```python
from build123d import *

# Parameters (mm, degrees)
F0_R     = 14.75
F1_DEPTH = 10
F3_DEPTH = 10


# Not quite as in the source:
# - a feature names something its author has since deleted; it is built from what else it names


with BuildPart() as f1:
    # F0 (on Top) → F1 (new body)
    with BuildSketch(Plane.XY):
        with BuildLine():
            ThreePointArc((0, 20), (5.8578643763, 5.8578643763), (20, 0))
            Line((20, 0), (97.5, 0))
            ThreePointArc((97.5, 0), (99.267766953, 0.732233047), (100, 2.5))
            Line((100, 2.5), (100, 37.5))
            ThreePointArc((100, 37.5), (99.267766953, 39.267766953), (97.5, 40))
            Line((97.5, 40), (20, 40))
            ThreePointArc((20, 40), (5.8578643763, 34.1421356237), (0, 20))
        make_face()
        with Locations((20, 20)):
            Circle(F0_R, mode=Mode.SUBTRACT)
    extrude(amount=F1_DEPTH)

    # F2 (on face) → F3 (join)
    with BuildSketch(Plane.XY.offset(10)):
        with BuildLine():
            ThreePointArc((22.5, 37.5), (21.767766953, 39.267766953), (20, 40))
            ThreePointArc((20, 40), (0, 20), (20, 0))
            ThreePointArc((20, 0), (21.767766953, 0.732233047), (22.5, 2.5))
            Line((22.5, 2.5), (22.5, 2.75))
            ThreePointArc((22.5, 2.75), (21.767766953, 4.517766953), (20, 5.25))
            ThreePointArc((20, 5.25), (5.25, 20), (20, 34.75))
            ThreePointArc((20, 34.75), (21.767766953, 35.482233047), (22.5, 37.25))
            Line((22.5, 37.25), (22.5, 37.5))
        make_face()
        with BuildLine():
            ThreePointArc((100, 37.5), (99.267766953, 39.267766953), (97.5, 40))
            ThreePointArc((97.5, 40), (95.732233047, 39.267766953), (95, 37.5))
            Line((95, 37.5), (95, 2.5))
            ThreePointArc((95, 2.5), (95.732233047, 0.732233047), (97.5, 0))
            ThreePointArc((97.5, 0), (99.267766953, 0.732233047), (100, 2.5))
            Line((100, 2.5), (100, 37.5))
        make_face()
    extrude(amount=F3_DEPTH)


solid = f1.part
```
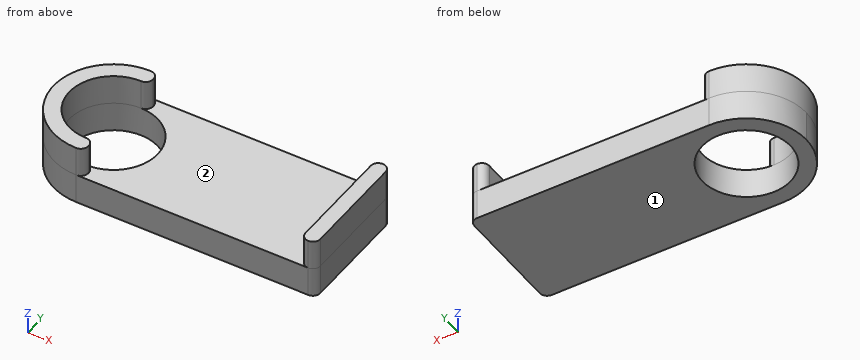
Design review of the part built by this model. Coordinates are the model's own, in mm. Face numbers are marked on the shaded views. Give positions to 0.01 mm unless a question says otherwise; leave off trailing zeros. Order: outer loops, then holes, each group sorted by start corner. A loop starts at its lowest first (then second) coordinate and runs counter-clockwise, first axis right, second up. Notation, with made-up numbers: (35, 18.25) - (79, 18.25) arc R16 cw to (79, 45.25) - close; hole circle Ø9 at (41.25, 71). An arc over 180 degrees is marked (long way). Use a Markdown table: item, result. Add a question column.
(1) Add section B-B on y = 27. Give the boundary of the cut face in (x, z) (3 decimals).
(2) Add section D-D on y = 15. Give the boundary of the cut face in (x, z), then the cut area to 3 significant figures.
(3) Add section A-A on z = 13. Give the boundary of the cut face in (x, y), then the cut area to 3 significant figures.
(4) Wall thickness on probe 1 along Y at (x, z) = (20, 4.5); probe 2 along X at (y, z) = (20, 4.25); probe 3 along Z at (x, y) = (82, 21): over which ranges is each line inside the solid? List them lowest first. Write a range as [from, to].
(5) Add section C-C on x = 37.5. Give the boundary of the cut face in (y, z).
(6) Clearance check with flat-ended pins moving along their axes: P1, Ø5, axis at y = 17, z = 15, coming from the -X side; P2, Ø8, axis at x = 52, z = 16, coming from the +Y side; P3, Ø12, axis at y = 29.5, z = 15.5, coming from the -X side; P4, Ø12, axis at x = 71.5, y = 21.5, coming from the +Z side. State where each tip first meets the part, or that it passes through.
(7) Mouldability with a two-part tool opening along X and no side actions: class the marked faces 1 and 2 as +X half, -X half, draft (parallel to the pull), parting line (faces both ways), or undercut.
Report:
| question | item | result |
|---|---|---|
| 1 | outline | (1.265, 0) - (7.017, 0) - (7.017, 20) - (1.265, 20) - close; (32.983, 0) - (100, 0) - (100, 20) - (95, 20) - (95, 10) - (32.983, 10) - close |
| 2 | outline | (0.64, 0) - (6.12, 0) - (6.12, 20) - (0.64, 20) - close; (33.88, 0) - (100, 0) - (100, 20) - (95, 20) - (95, 10) - (33.88, 10) - close |
| 2 | area | 821 mm² |
| 3 | outline | (20, 0) arc R2.5 ccw to (22.5, 2.5) - (22.5, 2.75) arc R2.5 ccw to (20, 5.25) arc R14.75 cw to (20, 34.75) arc R2.5 ccw to (22.5, 37.25) - (22.5, 37.5) arc R2.5 ccw to (20, 40) arc R20 ccw to start; (95, 2.5) arc R2.5 ccw to (100, 2.5) - (100, 37.5) arc R2.5 ccw to (95, 37.5) - close |
| 3 | area | 502 mm² |
| 4 | probe 1 | y = [0, 5.25], [34.75, 40] |
| 4 | probe 2 | x = [0, 5.25], [34.75, 100] |
| 4 | probe 3 | z = [0, 10] |
| 5 | outline | (0, 0) - (40, 0) - (40, 10) - (0, 10) - close |
| 6 | P1 | stops at x = 0.01 |
| 6 | P2 | passes through |
| 6 | P3 | stops at x = 0.31 |
| 6 | P4 | stops at z = 10 |
| 7 | face 1 | draft |
| 7 | face 2 | undercut |
